from build123d import *

# Parameters (mm, degrees)
CROQUIS1_W                 = 58.7375
CROQUIS1_H                 = 8.6614
SALIENTE_EXTRUIR1_DEPTH    = 4.7244
CORTAR_EXTRUIR2_DEPTH      = 60.560336732
CORTAR_EXTRUIR2_DEPTH_BACK = 60.560336732
CROQUIS2_W                 = 3.96875
CROQUIS2_H                 = 3.175
CORTAR_EXTRUIR4_DEPTH      = 60.560336732
SALIENTE_EXTRUIR2_DEPTH    = 8.6614


with BuildPart() as part:
    # Croquis1 → Saliente-Extruir1 (new body)
    with BuildSketch(Plane.XY):
        with Locations((29.36875, 4.3307)):
            Rectangle(CROQUIS1_W, CROQUIS1_H)
    extrude(amount=SALIENTE_EXTRUIR1_DEPTH)

    # Croquis2 → Cortar-Extruir2 (cut, two sides: drawn at the far end of the back side and taken through both)
    with BuildSketch(Plane.XY.offset(-CORTAR_EXTRUIR2_DEPTH_BACK)):
        with Locations((29.765625, 1.5875)):
            Rectangle(CROQUIS2_W, CROQUIS2_H)
    extrude(amount=CORTAR_EXTRUIR2_DEPTH + CORTAR_EXTRUIR2_DEPTH_BACK, mode=Mode.SUBTRACT)

    # Croquis4 → Cortar-Extruir4 (cut, through all)
    with BuildSketch(Plane(origin=(0, 8.6614, 0), x_dir=(1, 0, 0), z_dir=(0, 1, 0))):
        Polygon((0.5715, -4.7244), (0, -4.7244), (0, -2.223247059), align=None)
    extrude(amount=-CORTAR_EXTRUIR4_DEPTH, mode=Mode.SUBTRACT)

    # Croquis5 → Saliente-Extruir2 (add)
    with BuildSketch(Plane(origin=(0, 8.6614, 0), x_dir=(1, 0, 0), z_dir=(0, 1, 0))):
        Polygon((-0.6985, 0), (0.28575, 0), (0.5715, -4.7244), align=None)
    extrude(amount=-SALIENTE_EXTRUIR2_DEPTH)


solid = part.part
The model under review builds one solid part; all positions refer to its coordinate system, in mm. A direction names the side the tool comes from. Round coordinates to 2 decimals unless told otherwise and drop trailing zeros. Loops run counter-clockwise (first coordinate to the right, second up) from the corner with the lowest first, then second, coordinate; pieces in that order, holes last. Notation, with made-up numbers: (19, 19) -> (61, 19) arc R10 ccw to (61, 24) -> close; hole circle Ø5 at (-16, 4.25). An arc over 180 degrees is marked (long way). Answer as CSV lines item,"result".
1) For P1, Ø4, axis at x = 17.5, y = 1, coming from the -Z side; P2, Ø2, axis at x = 30, z = 2, coming from the -Y side (3 decimals); P3, Ø1.6, axis at y = 1.5, z = 2, coming from the -X side, all flat-tipped, find the tip position at first contact; note any pin that passes through.
Geometry results:
P1,"stops at z = 0"
P2,"stops at y = 3.175"
P3,"stops at x = -0.38"
2) To check wall thickness, follow line 1 along X through (y, z) = (1.25, 3.6); line 2 along X through (y, z) = (1, 3.3); line 3 along X through (y, z) = (3.25, 2.95). State the ranges of each line that lie inside material, in increasing order. Write a range as from..to.
Geometry results:
line 1,"x = 0.27..27.78, 31.75..58.74"
line 2,"x = 0.19..27.78, 31.75..58.74"
line 3,"x = 0.09..58.74"
3) Draft analysis for pull direction X (two halves, no side actions). For faces 1 (the face through (-0.055, 4.391, 2.395)), 2 (the face through (58.738, 4, 2)), 3 (the face through (29, 8.661, 2)), 4 (the face through (31.75, 2, 2)), state which applies: pulls with the +X half, pulls with the -X half, needs draft (parallel to the pull), parting line crosses it, or undercut.
Geometry results:
face 1,"pulls with the -X half"
face 2,"pulls with the +X half"
face 3,"needs draft"
face 4,"undercut"
4) Tool access review of faces 5 (the face through (29, 4, 0)), 6 (the face through (27.781, 2, 2)): name each direction out of +Z, -Z, +X, -X, +Y, -Y from which nothing blocks a thin tool from reaching the whole face with its end or side.
Geometry results:
face 5,"-Z, +X, -X, +Y, -Y"
face 6,"+Z, -Z, -Y"
5) Add section A-A on y = 2.25. Write out the cut boundary in (x, z), plus the area to 3 significant figures.
Geometry results:
outline,"(-0.7, 0) -> (27.78, 0) -> (27.78, 4.72) -> (0.57, 4.72) -> close; (31.75, 0) -> (58.74, 0) -> (58.74, 4.72) -> (31.75, 4.72) -> close"
area,"259 mm²"
